```python
from build123d import *

# Parameters (mm, degrees)
F1_DEPTH    = 20
F2_R        = 1.75
F3_DEPTH    = 40.001
F4_R        = 3
F5_DEPTH    = 7.5
F6_R        = 1.75
F7_DEPTH    = 15.001
F8_T1_DEPTH = 45
F10_DEPTH   = 2.5


# Not quite as in the source:
# - a fillet or chamfer that OpenCascade refuses, or shapes differently, is made with other operations: its cross-section is extruded or revolved along the edge and cut away or added


with BuildPart() as f1:
    # F0 (on Top) → F1 (new body)
    with BuildSketch(Plane.XY):
        Polygon((0, 15), (0, 0), (85, 0), (85, 40), (70, 40), (70, 15), align=None)
    extrude(amount=F1_DEPTH)

    # F2 (on face) → F3 (cut, through all)
    with BuildSketch(Plane.XZ):
        with Locations((7.5, 14.75)):
            Circle(F2_R)
        with Locations((7.5, 5.25)):
            Circle(F2_R)
    extrude(amount=-F3_DEPTH, mode=Mode.SUBTRACT)

    # F4 (on face) → F5 (cut)
    with BuildSketch(Plane.XZ):
        with Locations((7.5, 14.75)):
            Circle(F4_R)
        with Locations((7.5, 5.25)):
            Circle(F4_R)
    extrude(amount=-F5_DEPTH, mode=Mode.SUBTRACT)

    # F6 (on face) → F7 (cut, through all)
    with BuildSketch(Plane(origin=(70, 0, 0), x_dir=(0, -1, 0), z_dir=(-1, 0, 0))):
        with Locations((-27.5, 14.75)):
            Circle(F6_R)
        with Locations((-27.5, 5.25)):
            Circle(F6_R)
    extrude(amount=-F7_DEPTH, mode=Mode.SUBTRACT)

    # F8: fillet of radius 5 on 2 edges, made by hand

    # F8_s2 → F8_t1 (cut)
    with BuildSketch(Plane.XY.offset(-12.5)):
        with BuildLine():
            ThreePointArc((80, 0), (83.5355339059, 1.4644660941), (85, 5))
            Line((85, 5), (85, 0))
            Line((85, 0), (80, 0))
        make_face()
        with BuildLine():
            ThreePointArc((0, 5), (1.4644660941, 1.4644660941), (5, 0))
            Line((5, 0), (0, 0))
            Line((0, 0), (0, 5))
        make_face()
    extrude(amount=F8_T1_DEPTH, mode=Mode.SUBTRACT)

    # F9 (on face) → F10 (cut)
    with BuildSketch(Plane.YZ.offset(85)):
        Polygon((27.5, 11.5745735195), (30.25, 13.1622867597), (30.25, 16.3377132403), (27.5, 17.9254264805), (24.75, 16.3377132403), (24.75, 13.1622867597), align=None)
        Polygon((30.25, 6.8377132403), (27.5, 8.4254264805), (24.75, 6.8377132403), (24.75, 3.6622867597), (27.5, 2.0745735195), (30.25, 3.6622867597), align=None)
    extrude(amount=-F10_DEPTH, mode=Mode.SUBTRACT)


solid = f1.part
```
Can you work these out from the model? Positions are in its coordinate system, mm. A direction names the side the tool comes from. Round coordinates to 2 decimals unless told otherwise and drop trailing zeros. Order: outer loops, then holes, each group sorted by start corner. A loop starts at its lowest first (then second) coordinate and runs counter-clockwise, first axis right, second up. Notation, with made-up numbers: (53.5, 20.25) -> (69.5, 20.25) arc R30 cw to (69.5, 54.25) -> close; hole circle Ø4 at (-19.5, -34). An arc over 180 degrees is marked (long way). Return JSON: item names as keys, results as strings. Group by question number.
1. If we section it at B-B, the plane z = 14.75: Write out the boundary of the cut face in (x, y).
2. If we section it at A-A, the plane x = 7.5: Write out the boundary of the cut face in (y, z).
3. We'd pull the mould along Y, two halves only. Please class faces 1 (the face through (78, 40, 10)), 2 (the face through (8.31, 11.2, 3.7)), 3 (the face through (82.5, 26, 4)): released by +Y, released by -Y, zero draft, split by the parting line, or undercut.
4. If we section it at C-C, the plane z = 10: Write out the boundary of the cut face in (x, y), then the cut area to 3 significant figures.
5. I need wall thicknesses on line 1 (Z direction, x = 77.5, y = 27.5); line 2 (Z direction, x = 7.5, y = 3.25); line 3 (Y direction, x = 12, z = 6.75). Which ranges of each line are inside material? Lowest first, please. Write a range as [from, to].
6. Will these pins go through, and if not, where does the flat tip stop? pin 1 (6 mm diameter, centred on x = 49.5, z = 12, fed in from +Y); pin 2 (0.8 mm diameter, centred on x = 83.5, z = 5, fed in from -Y); pin 3 (1.6 mm diameter, centred on y = 28.5, z = 5.5, fed in from +X); pin 4 (3 mm diameter, centred on y = 27.5, z = 5.25, fed in from +X) (3 decimals).
7. If we section it at D-D, the plane x = 50: Write out the boundary of the cut face in (y, z).
8. Which directions (+Z, -Z, +X, -X, +Y, -Y) give clear straight access to the entire face, cutting with the end or side of a thin tool? Please do faces 4 (the face through (8.884, 3.698, 12.088)), 5 (the face through (84, 30.25, 15)), 6 (the face through (51, 11, 0)).
Output values:
{
 "1": {"outline": "(0, 5) arc R5 ccw to (4.5, 0.03) -> (4.5, 7.5) -> (5.75, 7.5) -> (5.75, 15) -> (0, 15) -> close; (9.25, 7.5) -> (10.5, 7.5) -> (10.5, 0) -> (80, 0) arc R5 ccw to (85, 5) -> (85, 24.75) -> (82.5, 24.75) -> (82.5, 25.75) -> (70, 25.75) -> (70, 15) -> (9.25, 15) -> close; (70, 29.25) -> (82.5, 29.25) -> (82.5, 30.25) -> (85, 30.25) -> (85, 40) -> (70, 40) -> close"},
 "2": {"outline": "(0, 0) -> (15, 0) -> (15, 3.5) -> (7.5, 3.5) -> (7.5, 2.25) -> (0, 2.25) -> close; (0, 8.25) -> (7.5, 8.25) -> (7.5, 7) -> (15, 7) -> (15, 13) -> (7.5, 13) -> (7.5, 11.75) -> (0, 11.75) -> close; (0, 17.75) -> (7.5, 17.75) -> (7.5, 16.5) -> (15, 16.5) -> (15, 20) -> (0, 20) -> close"},
 "3": {"face 1": "released by +Y", "face 2": "zero draft", "face 3": "undercut"},
 "4": {"outline": "(0, 5) arc R5 ccw to (5, 0) -> (80, 0) arc R5 ccw to (85, 5) -> (85, 40) -> (70, 40) -> (70, 15) -> (0, 15) -> close", "area": "1,640 mm²"},
 "5": {"line 1": "[0, 3.5], [7, 13], [16.5, 20]", "line 2": "[0, 2.25], [8.25, 11.75], [17.75, 20]", "line 3": "[0, 15]"},
 "6": {"pin 1": "y = 15", "pin 2": "y = 1.08", "pin 3": "x = 82.5", "pin 4": "through"},
 "7": {"outline": "(0, 0) -> (15, 0) -> (15, 20) -> (0, 20) -> close"},
 "8": {"face 4": "-Y", "face 5": "+X", "face 6": "-Z, +X, -X, +Y, -Y"}
}
